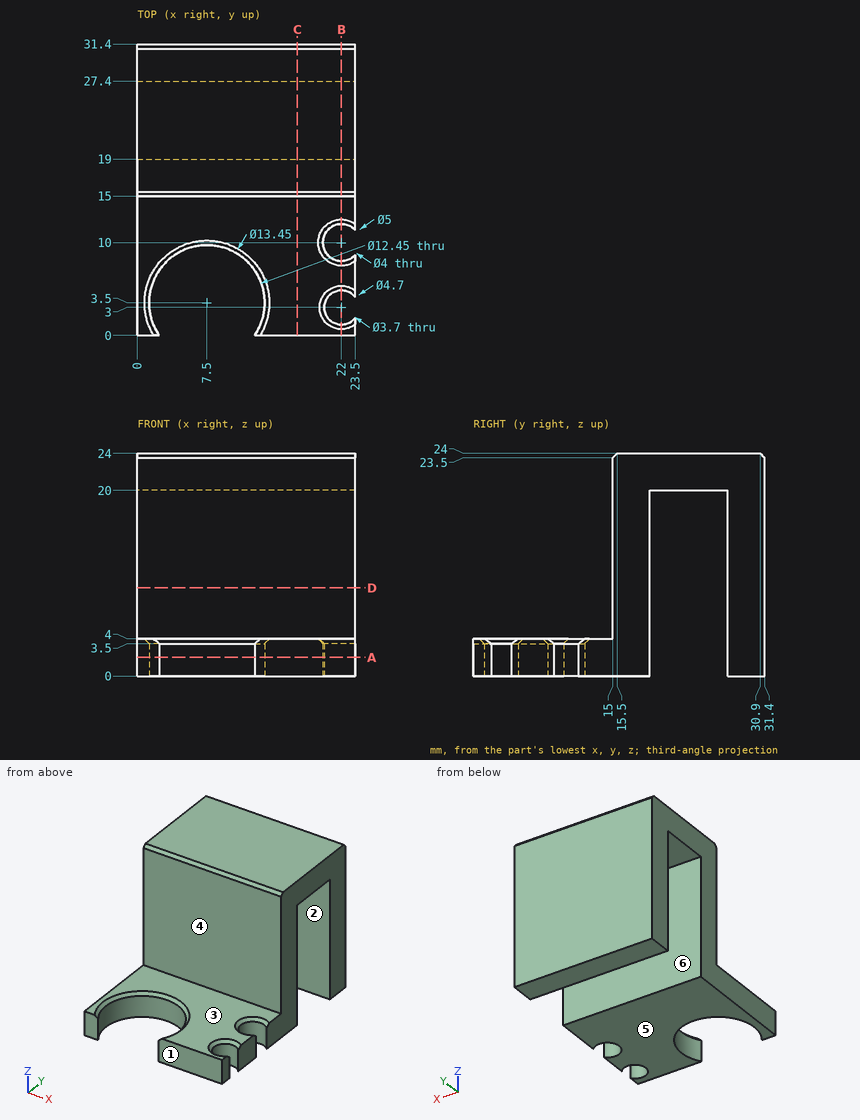
Source: three-view drawing plus pictorial views. Frame: mm from the lowest corner of the part. A direction names the side the tool comes from. Round coordinates to 2 decimals unless told otherwise and drop trailing zeros. Loops run counter-clockwise (first coordinate to the right, second up) from the corner with the lowest first, then second, coordinate; pieces in that order, holes last. Notation, with made-up numbers: M 87.25,-10 L 116.25,-10 A26 ccw 116.25,5 Z; hole C 38,33 d4. An arc over 180 degrees is marked long. Put each result on its own line as item: value. Start each with the question number.
(1) Section query D-D (z = 9.5). Return loops of the section in (x, y), then the cut area to 3 significant figures.
(2) Contact query for flat-ended pins moving along their axis: pin 1 Ø4 at (y, z) = (16.5, 20) entering from -X; pin 2 Ø1.5 at (x, y) = (12.5, 7) entering from +Z; pin 3 Ø2 at (x, z) = (18, 20) entering from -Y; pin 4 Ø6 at (x, z) = (6.5, 6) entering from -Y. Output: stop coordinate, or through.
(3) Section query C-C (x = 17.25). Return loops of the section in (y, z).
(4) Section query A-A (z = 2). Return loops of the section in (x, y) (3 decimals).
(5) Draft query along Y for the marked faces 1, 2 and 3. Return one class per face: +Y half, -Y half, draft (parallel to the pull), parting line (faces both ways), or undercut.
(6) Set-up query: the marked faces 4, 5 and 6. Return all of +Z, -Z, +X, -X, +Y, -Y with unobstructed straight access to the full face (end or side cutting, diameter ignored); none if empty.
(7) Material intervals for line 1 along Y through (x, z) = (22, 1.45); line 2 along Y through (x, z) = (22.75, 17); line 3 along Y through (x, z) = (7.5, 2.05) (3 decimals), sorted ascending. Write a range as [from, to].
(8) Section query B-B (x = 22). Return loops of the section in (y, z), then the cut area to 3 significant figures.
Findings below:
1. outline: M 0,15 L 23.5,15 L 23.5,19 L 0,19 Z; M 0,27.4 L 23.5,27.4 L 23.5,31.4 L 0,31.4 Z
1. area: 188 mm2
2. pin 1: stops at x = 0
2. pin 2: stops at z = 4
2. pin 3: stops at y = 15
2. pin 4: stops at y = 9.13
3. outline: M 0,0 L 19,0 L 19,20 L 27.4,20 L 27.4,0 L 31.4,0 L 31.4,23.5 L 30.9,24 L 15.5,24 L 15,23.5 L 15,4 L 0,4 Z
4. outline: M 0,0 L 2.352,0 A6.225 cw long 12.648,0 L 23.5,0 L 23.5,1.917 A1.85 cw long 23.5,4.083 L 23.5,8.677 A2 cw long 23.5,11.323 L 23.5,19 L 0,19 Z; M 0,27.4 L 23.5,27.4 L 23.5,31.4 L 0,31.4 Z
5. face 1: -Y half
5. face 2: undercut
5. face 3: draft
6. face 4: +Z, +X, -X, -Y
6. face 5: -Z, +X, -X, +Y, -Y
6. face 6: -Z, +X, -X
7. line 1: y = [0, 1.15], [4.85, 8], [12, 19], [27.4, 31.4]
7. line 2: y = [15, 19], [27.4, 31.4]
7. line 3: y = [9.725, 19], [27.4, 31.4]
8. outline: M 0,0 L 1.15,0 L 1.15,3.5 L 0.65,4 L 0,4 Z; M 4.85,0 L 8,0 L 8,3.5 L 7.5,4 L 5.35,4 L 4.85,3.5 Z; M 12,0 L 19,0 L 19,20 L 27.4,20 L 27.4,0 L 31.4,0 L 31.4,23.5 L 30.9,24 L 15.5,24 L 15,23.5 L 15,4 L 12.5,4 L 12,3.5 Z
8. area: 254 mm2
